Part model, mm, in its own coordinate system. A direction names the side the tool comes from. Give positions to 0.01 mm unless a question says otherwise; leave off trailing zeros. Order: outer loops, then holes, each group sorted by start corner. A loop starts at its lowest first (then second) coordinate and runs counter-clockwise, first axis right, second up. Notation, with made-up numbers: (73.25, 74.5) - (99.25, 74.5) arc R10 ccw to (99.25, 85.5) - close; hole circle Ø7 at (83.5, 60). An arc over 180 degrees is marked (long way). Use one line per item in the form item = value. Start each with the question number.
1. Pin check, flat tips, straight feed: P1, Ø6.5, axis at y = -1, z = 31.5, coming from the -X side; P2, Ø2, axis at y = 1, z = 55, coming from the +X side; P3, Ø2, axis at x = 68, y = -4, coming from the -Z side; P4, Ø9.5, axis at x = 10, z = 107.5, coming from the +Y side. Stop position of each tip, or through.
2. Pull direction Z, two halves, no side cores. Call faces 4 (the face through (85, -5, 65)), 5 (the face through (87.6, -4.9, 70.7)), 6 (the face through (50, 1, 65)), 7 (the face through (30, -4, 32)): +Z half, -Z half, draft (parallel to the pull), parting line (faces both ways), or undercut.
3. Band-saw the part on C-C, the plane y = -1.5. State how many separate pieces and enclosed holes the cut face has, plus the area to 3 significant figures.
4. Tool access for faces 1 (the face through (49, 0, 90)), 2 (the face through (70, -4, 32)), 3 (the face through (15, -5, 65)): list every direction of +Z, -Z, +X, -X, +Y, -Y with a clear straight run to the whole face (end or side of a thin tool).
5. Drill centre lines: line 1 (Z direction, x = 38, y = 2.25); line 2 (X direction, y = -5.75, z = 11); line 3 (Z direction, x = 50, y = -5.75). Where is each one in solid material? Low to high.
6. Band-saw the part on D-D, the plane z = 72.5. List the corners of the cut face in (x, y).
7. Band-saw the part on A-A, the plane x = 38. List the corners of the cut face in (y, z).
8. Band-saw the part on B-B, the plane z = 59. List the corners of the cut face in (x, y), plus the area to 3 significant figures.
from build123d import *

# Parameters (mm, degrees)
F0_R     = 3
F1_DEPTH = 10
F2_W     = 40
F2_H     = 65
F2_R     = 3
F3_DEPTH = 2.986


with BuildPart() as f1:
    # F0 (on Front) → F1 (new body)
    with BuildSketch(Plane.XZ):
        Polygon((30, 65), (30, 0), (70, 0), (70, 65), (100, 65), (100, 115), (0, 115), (0, 65), align=None)
        with Locations((38, 11)):
            Circle(F0_R, mode=Mode.SUBTRACT)
        with Locations((62, 11)):
            Circle(F0_R, mode=Mode.SUBTRACT)
        with Locations((10, 72.5)):
            Circle(F0_R, mode=Mode.SUBTRACT)
        with Locations((38, 59)):
            Circle(F0_R, mode=Mode.SUBTRACT)
        with Locations((10, 107.5)):
            Circle(F0_R, mode=Mode.SUBTRACT)
        with Locations((62, 59)):
            Circle(F0_R, mode=Mode.SUBTRACT)
        with Locations((50, 72.5)):
            Circle(F0_R, mode=Mode.SUBTRACT)
        with Locations((90, 72.5)):
            Circle(F0_R, mode=Mode.SUBTRACT)
        with Locations((50, 107.5)):
            Circle(F0_R, mode=Mode.SUBTRACT)
        with Locations((90, 107.5)):
            Circle(F0_R, mode=Mode.SUBTRACT)
    extrude(amount=F1_DEPTH)

    # F2 (on face) → F3 (join)
    with BuildSketch(Plane(origin=(0, 0, 0), x_dir=(-1, 0, 0), z_dir=(0, 1, 0))):
        with Locations((-50, 32.5)):
            Rectangle(F2_W, F2_H)
        with Locations((-62, 11)):
            Circle(F2_R, mode=Mode.SUBTRACT)
        with Locations((-38, 11)):
            Circle(F2_R, mode=Mode.SUBTRACT)
        with Locations((-62, 59)):
            Circle(F2_R, mode=Mode.SUBTRACT)
        with Locations((-38, 59)):
            Circle(F2_R, mode=Mode.SUBTRACT)
    extrude(amount=F3_DEPTH)


solid = f1.part
From the geometry:
q1.P1 = 30
q1.P2 = 70
q1.P3 = 0
q1.P4 = 0
q2.face_4 = -Z half
q2.face_5 = undercut
q2.face_6 = +Z half
q2.face_7 = draft
q3.separate_pieces = 1
q3.enclosed_holes = 10
q3.area = 7,320 mm²
q4.face_1 = +Z, +X, -X, +Y
q4.face_2 = -Z, +X, +Y, -Y
q4.face_3 = -Z, -X, +Y, -Y
q5.line_1 = 0 to 8, 14 to 56, 62 to 65
q5.line_2 = 30 to 35, 41 to 59, 65 to 70
q5.line_3 = 0 to 69.5, 75.5 to 104.5, 110.5 to 115
q6.outline = (0, -10) - (7, -10) - (7, 0) - (0, 0) - close; (13, -10) - (47, -10) - (47, 0) - (13, 0) - close; (53, -10) - (87, -10) - (87, 0) - (53, 0) - close; (93, -10) - (100, -10) - (100, 0) - (93, 0) - close
q7.outline = (-10, 0) - (2.99, 0) - (2.99, 8) - (-10, 8) - close; (-10, 14) - (2.99, 14) - (2.99, 56) - (-10, 56) - close; (-10, 62) - (2.99, 62) - (2.99, 65) - (0, 65) - (0, 115) - (-10, 115) - close
q8.outline = (30, -10) - (35, -10) - (35, 2.99) - (30, 2.99) - close; (41, -10) - (59, -10) - (59, 2.99) - (41, 2.99) - close; (65, -10) - (70, -10) - (70, 2.99) - (65, 2.99) - close
q8.area = 364 mm²
